The drawing under review shows one solid part. Ordinate dimensions are in mm from its lowest x, y, z. Coordinates: 2 decimals unless noted, no trailing zeros. Order: outer loops, then holes, each group sorted by start corner. A loop starts at its lowest first (then second) coordinate and runs counter-clockwise, first axis right, second up.
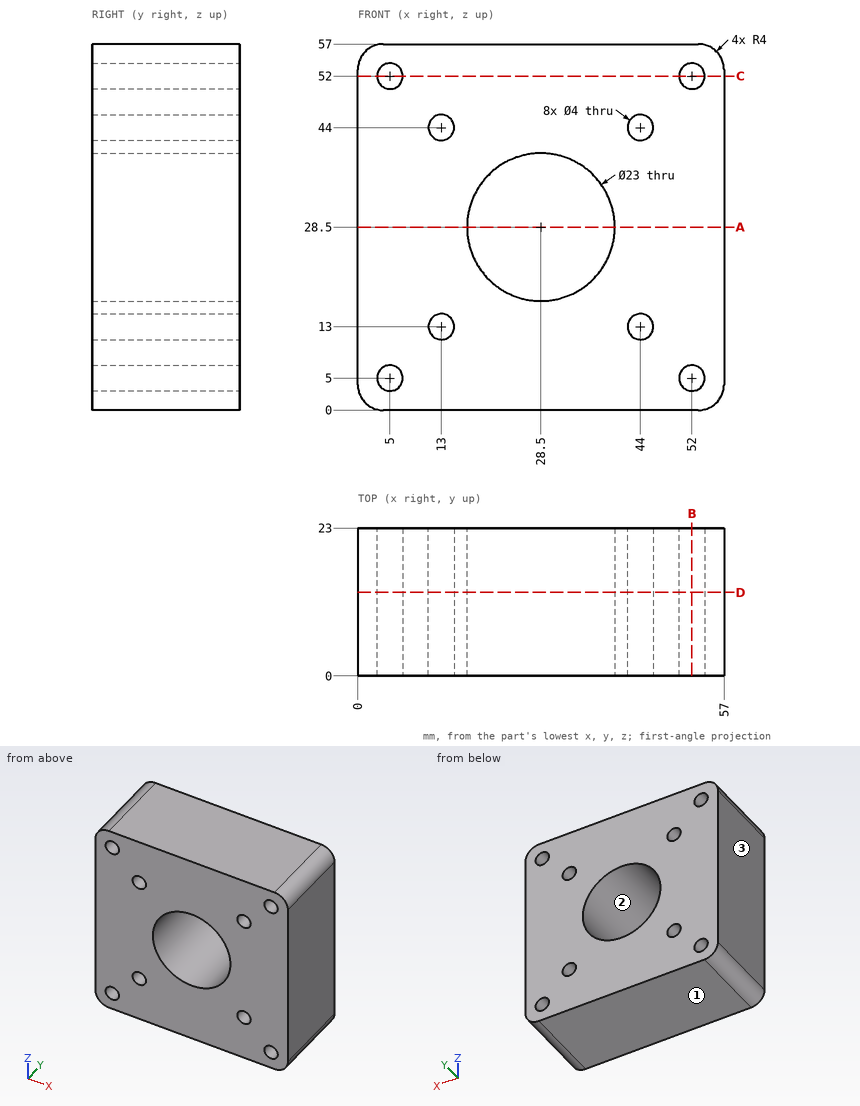
1. Take a section at A-A, the plane z = 28.5. Give the boundary of the cut face in (x, y).
Answer below:
outline: (0, 0) - (17, 0) - (17, 23) - (0, 23) - close; (40, 0) - (57, 0) - (57, 23) - (40, 23) - close
2. The part is to be moulded in two halves that separate along X. For the marked faces 1, 2 and 3, say which applies: +X half, -X half, draft (parallel to the pull), parting line (faces both ways), or undercut.
Answer below:
face 1: draft
face 2: undercut
face 3: -X half
3. Take a section at D-D, the plane y = 13. Give the number of separate pieces and of enclosed holes in the cut face, plus the area to 3 significant figures.
Answer below:
separate pieces: 1
enclosed holes: 9
area: 2,720 mm2
4. Take a section at B-B, the plane x = 52. Give the boundary of the cut face in (y, z).
Answer below:
outline: (0, 0) - (23, 0) - (23, 3) - (0, 3) - close; (0, 7) - (23, 7) - (23, 50) - (0, 50) - close; (0, 54) - (23, 54) - (23, 57) - (0, 57) - close
5. Take a section at C-C, the plane z = 52. Give the boundary of the cut face in (x, y).
Answer below:
outline: (0, 0) - (3, 0) - (3, 23) - (0, 23) - close; (7, 0) - (50, 0) - (50, 23) - (7, 23) - close; (54, 0) - (57, 0) - (57, 23) - (54, 23) - close
6. Clearance check with flat-ended pins moving along their axes: pin 1 Ø3 at (x, z) = (37, 32) entering from -Y; pin 2 Ø5 at (x, z) = (52, 52) entering from +Y. State where each tip first meets the part, or that it passes through.
Answer below:
pin 1: passes through
pin 2: stops at y = 23
7. To check wall thickness, follow L1, parallel to Z at x = 44, y = 12.5; L2, parallel to Z at x = 52, y = 6.75; L3, parallel to X at y = 17.25, z = 53. State the ranges of each line that lie inside material, in increasing order.
Answer below:
L1: z = 0 to 11, 15 to 42, 46 to 57
L2: z = 0 to 3, 7 to 50, 54 to 57
L3: x = 0 to 3.27, 6.73 to 50.27, 53.73 to 57
